```python
from build123d import *

# Parameters (mm, degrees)
F0_W     = 20
F0_H     = 5
F1_DEPTH = 1


with BuildPart() as f1:
    # F0 (on Top) → F1 (new body)
    with BuildSketch(Plane.XY):
        with Locations((-10, 2.5)):
            Rectangle(F0_W, F0_H)
        with Locations((10, 2.5)):
            Rectangle(F0_W, F0_H)
        Polygon((-20, 5), (0, 5), (-19.938792, 24.938792), align=None)
        Polygon((19.938792, 24.938792), (0, 5), (20, 5), align=None)
    extrude(amount=F1_DEPTH)


solid = f1.part
```
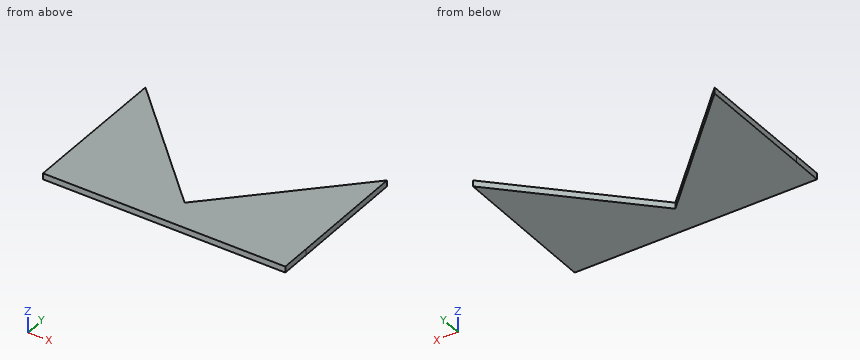
The model under review builds one solid part; all positions refer to its coordinate system, in mm. Round coordinates to 2 decimals unless told otherwise and drop trailing zeros. Loops run counter-clockwise (first coordinate to the right, second up) from the corner with the lowest first, then second, coordinate; pieces in that order, holes last. Notation, with made-up numbers: (-22.5, 26.5) - (16.5, 26.5) arc R20 cw to (16.5, 33.5) - close; hole circle Ø6 at (72, -5.5). An arc over 180 degrees is marked (long way). Use a Markdown table: item, result. Add a question column.
Q1. Add section C-C (x = 13.5). State the section outline as (y, z) points, plus the area to 3 significant figures.
Q2. Add section B-B (y = 7.75). State the section outline as (x, z) points.
Q3. Add section D-D (y = 20.75). State the section outline as (x, z) points.
Q4. Add section A-A (z = 0.3). State the section outline as (x, y) points.
Q5. For probe 1 along X at (y, z) = (23.5, 0.9); probe 2 along X at (y, z) = (17, 0.1); probe 3 along Y at (x, z) = (15, 0.3), list the stretches that pass through material, from the lowest coordinate up.
Worked answers:
| question | item | result |
|---|---|---|
| 1 | outline | (0, 0) - (18.5, 0) - (18.5, 1) - (0, 1) - close |
| 1 | area | 18.5 mm² |
| 2 | outline | (-19.99, 0) - (-2.75, 0) - (-2.75, 1) - (-19.99, 1) - close; (2.75, 0) - (19.99, 0) - (19.99, 1) - (2.75, 1) - close |
| 3 | outline | (-19.95, 0) - (-15.75, 0) - (-15.75, 1) - (-19.95, 1) - close; (15.75, 0) - (19.95, 0) - (19.95, 1) - (15.75, 1) - close |
| 4 | outline | (-20, 0) - (20, 0) - (20, 5) - (19.94, 24.94) - (0, 5) - (-19.94, 24.94) - (-20, 5) - close |
| 5 | probe 1 | -19.94 to -18.5, 18.5 to 19.94 |
| 5 | probe 2 | -19.96 to -12, 12 to 19.96 |
| 5 | probe 3 | 0 to 20 |
